Part model, mm, in its own coordinate system. A direction names the side the tool comes from. Coordinates: 2 decimals unless noted, no trailing zeros. Order: outer loops, then holes, each group sorted by start corner. A loop starts at its lowest first (then second) coordinate and runs counter-clockwise, first axis right, second up. Notation, with made-up numbers: (62, -29) - (99, -29) arc R12 cw to (99, -22) - close; hole circle Ø6 at (-30.75, 60.5). An arc over 180 degrees is marked (long way). Use a Markdown table: item, result. Add a question column.
1) Two-plate mould, pull along Z, no slides. Class faces 1 (the face through (24, 5, 23)), 2 (the face through (10, 8, 0)), 3 (the face through (10.564, 4.93, 17.307)), 4 (the face through (5, 13, 10)): +Z half, -Z half, draft (parallel to the pull), parting line (faces both ways), or undercut.
2) Saw through at B-B on z = 15. List the corners of the cut face in (x, y), then the cut area to 3 significant figures.
3) Saw through at A-A on x = 15. List the corners of the cut face in (y, z).
4) Tool access for faces 5 (the face through (0, 8, 10)), 6 (the face through (20, 12, 2)), 7 (the face through (11, 14, 5)): list every direction of +Z, -Z, +X, -X, +Y, -Y with a clear straight run to the whole face (end or side of a thin tool).
5) Wall check: L1, parallel to Z at x = 14.75, y = 6; L2, parallel to Y at x = 10.5, z = 6; L3, parallel to X at y = 7.75, z = 15. Give the ranges that are in metal, low to high. Write a range as [from, to].
6) Saw through at D-D on y = 6.5. List the corners of the cut face in (x, z), then the cut area to 3 significant figures.
7) Drop flat-ended pins along their axis: P1, Ø5, axis at x = 6, z = 3, coming from the -Y side; P2, Ø5.5, axis at x = 13.5, z = 1.5, coming from the +Y side; P3, Ø5, axis at x = 16, y = 13.5, coming from the +Z side; P4, Ø5.5, axis at y = 13, z = 3.5, coming from the +X side. Give the stop position or say it passes through.
8) Saw through at C-C on y = 17. List the corners of the cut face in (x, z).
```python
from build123d import *

# Parameters (mm, degrees)
SKETCH_1_R      = 5
EXTRUDE_1_DEPTH = 10
SKETCH_2_W      = 10
SKETCH_2_H      = 5
EXTRUDE_2_DEPTH = 5
EXTRUDE_3_DEPTH = 5


with BuildPart() as part:
    # 草圖1 → 填料-伸長1 (new body)
    with BuildSketch(Plane(origin=(0, 0, 0), x_dir=(1, 0, 0), z_dir=(0, 1, 0))):
        with BuildLine():
            Line((0, 0), (25, 0))
            Line((25, 0), (25, -20))
            ThreePointArc((25, -20), (23.535533906, -23.535533906), (20, -25))
            Line((20, -25), (0, -25))
            Line((0, -25), (0, 0))
        make_face()
        with Locations(Location((15, -15, 0), (0, 0, 270))):
            Circle(SKETCH_1_R, mode=Mode.SUBTRACT)
    extrude(amount=EXTRUDE_1_DEPTH)

    # 草圖2 → 填料-伸長2 (add)
    with BuildSketch(Plane(origin=(0, 0, 0), x_dir=(-1, 0, 0), z_dir=(0, 0, -1))):
        Polygon((-10, 10), (0, 10), (0, 20), (-10, 20), (-10, 15), align=None)
        with Locations((-15, 12.5)):
            Rectangle(SKETCH_2_W, SKETCH_2_H)
    extrude(amount=-EXTRUDE_2_DEPTH)

    # 草圖3 → 填料-伸長3 (add)
    with BuildSketch(Plane.ZY):
        Polygon((5, 20), (5, 10), (25, 10), align=None)
    extrude(amount=-EXTRUDE_3_DEPTH)


solid = part.part
```
Results are:
| question | item | result |
|---|---|---|
| 1 | face 1 | +Z half |
| 1 | face 2 | -Z half |
| 1 | face 3 | undercut |
| 1 | face 4 | draft |
| 2 | outline | (0, 0) - (10, 0) - (10, 10) - (5, 10) - (5, 15) - (0, 15) - close; (20, 0) - (25, 0) - (25, 10) - (20, 10) - close |
| 2 | area | 175 mm2 |
| 3 | outline | (0, 0) - (15, 0) - (15, 5) - (10, 5) - (10, 10) - (0, 10) - close; (0, 20) - (10, 20) - (10, 25) - (0, 25) - close |
| 4 | face 5 | +Z, -Z, -X, +Y, -Y |
| 4 | face 6 | +Z, -Z, +X, +Y |
| 4 | face 7 | +Z, +X, +Y |
| 5 | L1 | [0, 10.01], [19.99, 25] |
| 5 | L2 | [0, 10] |
| 5 | L3 | [0, 10], [20, 25] |
| 6 | outline | (0, 0) - (25, 0) - (25, 20) arc R5 ccw to (20, 25) - (0, 25) - close; hole circle Ø10 at (15, 15) |
| 6 | area | 541 mm2 |
| 7 | P1 | y = 0 |
| 7 | P2 | y = 15 |
| 7 | P3 | z = 5 |
| 7 | P4 | x = 20 |
| 8 | outline | (0, 0) - (10, 0) - (10, 5) - (5, 5) - (5, 11) - (0, 11) - close |
